```python
from build123d import *

# Parameters (mm, degrees)
SKETCH1_W                 = 60
SKETCH1_H                 = 12.7
BOSS_EXTRUDE1_DEPTH       = 38
M8X1_0_TAPPED_HOLE1_D     = 7
M8X1_0_TAPPED_HOLE1_DEPTH = 19.05
M8X1_0_TAPPED_HOLE1_TIP   = 2.103012167
BOSS_EXTRUDE3_DEPTH       = 12.7
M4X0_7_TAPPED_HOLE1_D     = 3.3


with BuildPart() as part:
    # Sketch1 → Boss-Extrude1 (new body)
    with BuildSketch(Plane(origin=(0, 0, 0), x_dir=(1, 0, 0), z_dir=(0, 1, 0))):
        with Locations((-30, 6.35)):
            Rectangle(SKETCH1_W, SKETCH1_H)
    extrude(amount=BOSS_EXTRUDE1_DEPTH)

    # M8x1.0 Tapped Hole1
    with Locations(Plane(origin=(-30, 7.5, 0), x_dir=(1, 0, 0), z_dir=(0, 0, 1))):
        with Locations((0, 0)):
            Hole(M8X1_0_TAPPED_HOLE1_D / 2, depth=M8X1_0_TAPPED_HOLE1_DEPTH)
            with Locations((0, 0, -(M8X1_0_TAPPED_HOLE1_DEPTH + M8X1_0_TAPPED_HOLE1_TIP / 2))):  # 118° drill point
                Cone(0, M8X1_0_TAPPED_HOLE1_D / 2, M8X1_0_TAPPED_HOLE1_TIP, mode=Mode.SUBTRACT)

    # Sketch7 → Boss-Extrude3 (add)
    with BuildSketch(Plane.XY):
        Polygon((-60, 7.5), (-60, 10), (-65, 10), (-65, 5), (-60, 5), align=None)
        Polygon((5, 5), (0, 5), (0, 7.5), (0, 10), (5, 10), align=None)
    extrude(amount=-BOSS_EXTRUDE3_DEPTH)

    # M4x0.7 Tapped Hole1 (through all)
    with Locations(Plane(origin=(-52, 34.825, 0), x_dir=(1, 0, 0), z_dir=(0, 0, 1))):
        with Locations((0, 0), (22, 0), (44, 0)):
            Hole(M4X0_7_TAPPED_HOLE1_D / 2)


solid = part.part
```
Verification items for the finished model (mm, model axes). A direction names the side the tool comes from. Round coordinates to 2 decimals unless told otherwise and drop trailing zeros. Order: outer loops, then holes, each group sorted by start corner. A loop starts at its lowest first (then second) coordinate and runs counter-clockwise, first axis right, second up. Notation, with made-up numbers: (19.25, 87.5) -> (27.25, 87.5) arc R24 ccw to (27.25, 111.5) -> close; hole circle Ø1 at (-9.5, 83.25). An arc over 180 degrees is marked (long way). Put each result on its own line as item: value. Start each with the question number.
(1) Tool access check on faces 1 (the face through (2, 10, -6)), 2 (the face through (0, 2, -6)), 3 (the face through (-60, 2, -6)). Record the directions out of +Z, -Z, +X, -X, +Y, -Y that give a thin tool (end or side, any length) a straight path to the whole face; none if there is none.
(2) Draft check along Y on faces 4 (the face through (-50.35, 34.9, -6.44)), 5 (the face through (-31.615, 4.395, -6.439)), 6 (the face through (-30, 19, 0)), 7 (the face through (-63, 5, -6)). Enter one of: +Y half, -Y half, draft (parallel to the pull), parting line (faces both ways), or undercut.
(3) Section check B-B (y = 7.5). Enter the section's corners in (x, z).
(4) Depth check by flat-ended pin: pin 1 Ø3 at (x, y) = (-8, 34.825) entering from +Z; pin 2 Ø1.5 at (x, z) = (2, -9.5) entering from +Y; pin 3 Ø1.5 at (y, z) = (18.5, -2) entering from +X; pin 4 Ø4 at (x, z) = (-62.5, -6) entering from -Y. Enter the tip coordinate at first touch or a pass-through.
(5) Section check A-A (x = -52). Enter the section's corners in (y, z) (3 decimals), then the cut area to 3 significant figures.
(6) Material ranges on line 1 along X through (y, z) = (35, -7); line 2 along Y through (x, z) = (-8, -5) (3 decimals); line 3 along Y through (x, z) = (-30, -3.75) (3 decimals), recorded low to high.
(7) Section check D-D (z = -8.25). Enter the section's corners in (x, y) (3 decimals).
(8) Section check C-C (x = -30). Enter the section's corners in (y, z) (3 decimals), then the cut area to 3 significant figures.
Completed:
1. face 1: +Z, -Z, +X, +Y
1. face 2: +Z, -Z, +X, -Y
1. face 3: +Z, -Z, -X, -Y
2. face 4: undercut
2. face 5: undercut
2. face 6: draft
2. face 7: -Y half
3. outline: (-65, -12.7) -> (-33.5, -12.7) -> (-33.5, 0) -> (-65, 0) -> close; (-26.5, -12.7) -> (5, -12.7) -> (5, 0) -> (-26.5, 0) -> close
4. pin 1: passes through
4. pin 2: stops at y = 10
4. pin 3: stops at x = 0
4. pin 4: stops at y = 5
5. outline: (0, -12.7) -> (33.175, -12.7) -> (33.175, 0) -> (0, 0) -> close; (36.475, -12.7) -> (38, -12.7) -> (38, 0) -> (36.475, 0) -> close
5. area: 441 mm2
6. line 1: x = -60 to -53.64, -50.36 to -31.64, -28.36 to -9.64, -6.36 to 0
6. line 2: y = 0 to 33.175, 36.475 to 38
6. line 3: y = 0 to 4, 11 to 33.175, 36.475 to 38
7. outline: (-65, 5) -> (-60, 5) -> (-60, 0) -> (0, 0) -> (0, 5) -> (5, 5) -> (5, 10) -> (0, 10) -> (0, 38) -> (-60, 38) -> (-60, 10) -> (-65, 10) -> close; hole circle Ø3.3 at (-52, 34.825); hole circle Ø7 at (-30, 7.5); hole circle Ø3.3 at (-30, 34.825); hole circle Ø3.3 at (-8, 34.825)
8. outline: (0, -12.7) -> (4, -12.7) -> (4, 0) -> (0, 0) -> close; (11, -12.7) -> (33.175, -12.7) -> (33.175, 0) -> (11, 0) -> close; (36.475, -12.7) -> (38, -12.7) -> (38, 0) -> (36.475, 0) -> close
8. area: 352 mm2
